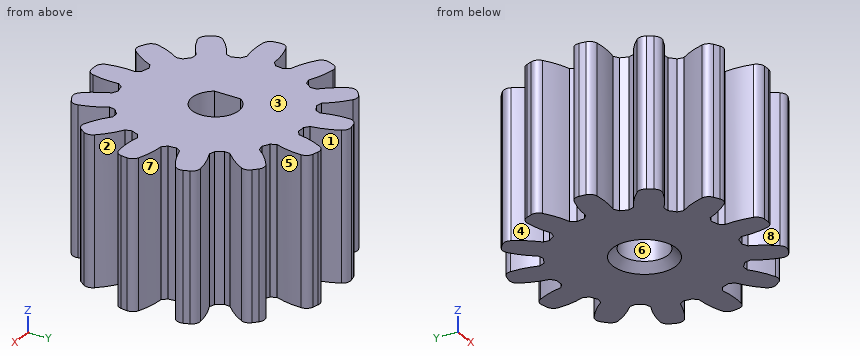
```python
from build123d import *

# Parameters (mm, degrees)
SKETCH1_R           = 15
BOSS_EXTRUDE1_DEPTH = 9
CUT_EXTRUDE1_DEPTH  = 24.043437244
CIRPATTERN1_COUNT   = 13
FILLET1_R           = 1
SKETCH3_R           = 2.85
CUT_EXTRUDE2_DEPTH  = 24
BOSS_EXTRUDE2_DEPTH = 8.5
FILLET3_R           = 1
CHAMFER2_SIZE       = 1


with BuildPart() as part:
    # Sketch1 → Boss-Extrude1 (new, symmetric)
    with BuildSketch(Plane.XY):
        Circle(SKETCH1_R)
    extrude(amount=BOSS_EXTRUDE1_DEPTH, both=True)

    # Sketch2 → Cut-Extrude1 (cut, symmetric)
    with BuildSketch(Plane.XY):
        with BuildLine():
            Line((2.488704723, 14.792104272), (2.488704723, 15.173999235))
            Line((2.488704723, 15.173999235), (-2.614354336, 15.173999235))
            Line((-2.614354336, 15.173999235), (-2.488704723, 14.792104272))
            ThreePointArc((-2.488704723, 14.792104272), (-1.497391845, 12.707607266), (-1.01110734, 10.451203852))
            ThreePointArc((-1.01110734, 10.451203852), (0, 10.5), (1.01110734, 10.451203852))
            ThreePointArc((1.01110734, 10.451203852), (1.497391845, 12.707607266), (2.488704723, 14.792104272))
        make_face()
    cut_extrude1 = extrude(amount=CUT_EXTRUDE1_DEPTH, both=True, mode=Mode.SUBTRACT)

    # CirPattern1: Cut-Extrude1 ×13 about axis
    cirpattern1_axis = Axis((0, 0, 0), (0, 0, 1))
    for i in range(1, CIRPATTERN1_COUNT):
        add(cut_extrude1.rotate(cirpattern1_axis, i * 360 / CIRPATTERN1_COUNT), mode=Mode.SUBTRACT)

    # Fillet1
    fillet1_edges = [part.edges().sort_by_distance(p)[0] for p in [
        (11.67180174, -9.421732544, 0),
        (7.946157272, -12.722365527, 0),
        (14.713364615, -2.918373125, 0),
        (-2.488704723, 14.792104272, 0),
        (12.948350901, -7.572331804, 0),
        (5.956369747, -13.766686582, 0),
        (1.123594773, -14.95785863, 0),
        (2.488704723, 14.792104272, 0),
        (-1.123594773, -14.95785863, 0),
        (-5.956369747, -13.766686582, 0),
        (-12.948350901, -7.572331804, 0),
        (-14.713364615, -2.918373125, 0),
        (-7.946157272, -12.722365527, 0),
        (-11.67180174, -9.421732544, 0),
        (-9.077872212, 11.941199107, 0),
        (-4.670595026, 14.254316613, 0),
        (-13.587408577, 6.354709133, 0),
        (-10.759917741, 10.451036801, 0),
        (-14.984233383, -0.68756812, 0),
        (-14.384272972, 4.253550406, 0),
        (4.670595026, 14.254316613, 0),
        (9.077872212, 11.941199107, 0),
        (10.759917741, 10.451036801, 0),
        (13.587408577, 6.354709133, 0),
        (14.384272972, 4.253550406, 0),
        (14.984233383, -0.68756812, 0),
    ]]
    fillet(fillet1_edges, radius=FILLET1_R)

    # Chamfer1
    # the kernel refuses this chamfer: 0.5 mm, written as the material it adds along each edge
    with BuildSketch(Plane(origin=(7.687254792, -7.152350227, 9), x_dir=(-0.6988462718759633, -0.7152718981513725, 0), z_dir=(0, 0, -1)), Plane(origin=(3.482863191, -9.905537037, 9), x_dir=(-0.9512010678205252, -0.3085717559613855, 0), z_dir=(0, 0, -1)), Plane(origin=(-1.519410394, -10.389484687, 9), x_dir=(-0.9856471623429421, 0.16881845682657493, 0), z_dir=(0, 0, -1)), Plane(origin=(-9.413501753, -4.651449748, 9), x_dir=(-0.42097653940929197, 0.9070715259928386, 0), z_dir=(0, 0, -1)), Plane(origin=(-6.173605368, -8.493326601, 9), x_dir=(-0.7942933703085662, 0.6075343956385179, 0), z_dir=(0, 0, -1)), Plane(origin=(-10.496878331, 0.256018188, 9), x_dir=(0.048780943351376956, 0.998809501139106, 0), z_dir=(0, 0, -1))) as chamfer1_piece_1:
        with BuildLine():
            Line((0.512668458, 0), (-0.025719054, -0.512719416))
            ThreePointArc((-0.025719054, -0.512719416), (-0.009930751, -0.26377362), (0, 0))
            ThreePointArc((0, 0), (0.263582733, -0.00312688), (0.512668458, 0))
        make_face()
    extrude(amount=18)
    with BuildSketch(Plane(origin=(6.173605368, -8.493326601, 9), x_dir=(0.5669781411868423, -0.8237328374031918, 0), z_dir=(0, 0, -1)), Plane(origin=(9.413501753, -4.651449748, 9), x_dir=(0.8848419486421701, -0.4658913241552447, 0), z_dir=(0, 0, -1)), Plane(origin=(1.519410394, -10.389484687, 9), x_dir=(0.11922647441292282, -0.9928670846589006, 0), z_dir=(0, 0, -1)), Plane(origin=(-3.482863191, -9.905537037, 9), x_dir=(-0.3558385408142222, -0.934547448164728, 0), z_dir=(0, 0, -1)), Plane(origin=(-10.130588961, -2.760646175, 9), x_dir=(-0.971256802316475, -0.23803408149669583, 0), z_dir=(0, 0, -1)), Plane(origin=(-7.687254792, -7.152350227, 9), x_dir=(-0.7493852346601237, -0.6621342538136743, 0), z_dir=(0, 0, -1)), Plane(origin=(-10.253127286, 2.263488646, 9), x_dir=(-0.9706251414754602, 0.24059683026952544, 0), z_dir=(0, 0, -1))) as chamfer1_piece_2:
        with BuildLine():
            Line((0.513364071, 0), (-0.025684204, -0.512024677))
            ThreePointArc((-0.025684204, -0.512024677), (-0.010082291, -0.263408394), (0, 0))
            ThreePointArc((0, 0), (0.263939908, -0.003296528), (0.513364071, 0))
        make_face()
    extrude(amount=18)
    with BuildSketch(Plane(origin=(-1.01110734, 10.451203852, 9), x_dir=(-0.12184667616261032, 0.9925489345660113, 0), z_dir=(0, 0, -1)), Plane(origin=(10.130588961, -2.760646175, 9), x_dir=(0.9712568023164747, -0.2380340814966975, 0), z_dir=(0, 0, -1)), Plane(origin=(-5.752207693, 8.784196415, 9), x_dir=(-0.569150362894187, 0.822233461017864, 0), z_dir=(0, 0, -1)), Plane(origin=(-9.175546584, 5.104835441, 9), x_dir=(-0.8860685604921126, 0.46355421053792145, 0), z_dir=(0, 0, -1)), Plane(origin=(3.961625519, 9.723966436, 9), x_dir=(0.35337061566617867, 0.9354834087164272, 0), z_dir=(0, 0, -1)), Plane(origin=(8.026797714, 6.769085497, 9), x_dir=(0.7476349580234212, 0.664109907727115, 0), z_dir=(0, 0, -1)), Plane(origin=(10.253127286, 2.263488646, 9), x_dir=(0.9706251414754612, 0.24059683026952128, 0), z_dir=(0, 0, -1))) as chamfer1_piece_3:
        with BuildLine():
            Line((0.513364071, 0), (-0.025684204, 0.512024677))
            ThreePointArc((-0.025684204, 0.512024677), (-0.010082291, 0.263408394), (0, 0))
            ThreePointArc((0, 0), (0.263939908, 0.003296528), (0.513364071, 0))
        make_face()
    extrude(amount=18)
    with BuildSketch(Plane(origin=(1.01110734, 10.451203852, 9), x_dir=(-0.9974069482855394, 0.07196790612298887, 0), z_dir=(0, 0, -1)), Plane(origin=(-3.961625519, 9.723966436, 9), x_dir=(-0.916605146006636, -0.39979370469550085, 0), z_dir=(0, 0, -1)), Plane(origin=(-8.026797714, 6.769085497, 9), x_dir=(-0.6258201510670891, -0.7799673958047002, 0), z_dir=(0, 0, -1)), Plane(origin=(5.752207693, 8.784196415, 9), x_dir=(-0.8497148387689841, 0.5272425369560002, 0), z_dir=(0, 0, -1)), Plane(origin=(9.175546584, 5.104835441, 9), x_dir=(-0.5073632998643495, 0.8617322565337555, 0), z_dir=(0, 0, -1)), Plane(origin=(10.496878331, 0.256018188, 9), x_dir=(-0.04878094335137992, 0.9988095011391058, 0), z_dir=(0, 0, -1))) as chamfer1_piece_4:
        with BuildLine():
            Line((0.512668458, 0), (-0.025719054, 0.512719416))
            ThreePointArc((-0.025719054, 0.512719416), (-0.009930751, 0.26377362), (0, 0))
            ThreePointArc((0, 0), (0.263582733, 0.00312688), (0.512668458, 0))
        make_face()
    extrude(amount=18)

    # Sketch3 → Cut-Extrude2 (cut)
    with BuildSketch(Plane(origin=(0, 0, -9), x_dir=(-1, 0, 0), z_dir=(0, 0, -1))):
        Circle(SKETCH3_R)
    extrude(amount=-CUT_EXTRUDE2_DEPTH, mode=Mode.SUBTRACT)

    # Sketch5 → Boss-Extrude2 (add)
    with BuildSketch(Plane.XY.offset(9)):
        Polygon((-2.35, 0), (-2.35, 1.61245155), (-2.85, 1.61245155), (-2.85, -1.61245155), (-2.35, -1.61245155), align=None)
    extrude(amount=-BOSS_EXTRUDE2_DEPTH)

    # Fillet3
    # the kernel refuses this fillet: 1 mm, written as the material it takes off along each edge
    with BuildSketch(Plane(origin=(-2.35, -4.11245155, 0.5), x_dir=(-1, 0, 0), z_dir=(0, 1, 0))) as fillet3_piece_1_section:
        with BuildLine():
            CenterArc((FILLET3_R, FILLET3_R), FILLET3_R, 180, 90)
            Line((0, FILLET3_R), (0, 0))
            Line((0, 0), (FILLET3_R, 0))
        make_face()
    fillet3_piece_1 = extrude(amount=8.224903099, mode=Mode.PRIVATE)
    fillet3_piece_1 = fillet3_piece_1 & Plane(origin=(0, 0, 0.5), x_dir=(-1, 0, 0), z_dir=(0, 0, -1)) * Cylinder(2.85, 21, mode=Mode.PRIVATE)
    add(fillet3_piece_1, mode=Mode.SUBTRACT)

    # Chamfer2
    chamfer2_edges = [part.edges().sort_by_distance(p)[0] for p in [
        (2.85, 0, -9),
    ]]
    chamfer(chamfer2_edges, length=CHAMFER2_SIZE)


solid = part.part
```
Read the model definition and answer for the solid it produces. Units are mm, in the model's axes. Face numbers are marked on the shaded views. A direction names the side the tool comes from. Give positions to 0.01 mm unless a question says otherwise; leave off trailing zeros. Order: outer loops, then holes, each group sorted by start corner. A loop starts at its lowest first (then second) coordinate and runs counter-clockwise, first axis right, second up.
(1) Straight lines are drawn through the part: L1, parallel to Y at x = -12.5, z = 4.5; L2, parallel to X at y = -10.5, z = 0.5; L3, parallel to X at y = 9.5, z = -1.5. For each, find the intervals that lie inside material, in ascending order.
(2) For the marked faces 4, 5, 6, 7 and 8, determine the directions among +Z, -Z, +X, -X, +Y, -Y from which every point of the face is accessible in a straight line to the end or side of a thin tool.
(3) Find section A-A (x = 0). Give the vertices of the cut face in (y, z).
(4) For a pull along Y with two mould halves and no side action, classify the marked faces 1, 2 and 3 as released by +Y, released by -Y, zero draft, split by the parting line, or undercut.
(5) Given pin 1 (4.5 mm diameter, centred on x = 0, y = 0, fed in from +Z); pin 2 (10 mm diameter, centred on y = 6.5, z = 4.5, fed in from +X); pin 3 (1.5 mm diameter, centred on x = -6, z = -7, fed in from +Y), each flat-ended and moving along its own axis, determine where each tip first touches the part or whether it passes through.
Result sheet:
1. L1: y = -8.29 to -7.02, -3.11 to 0.1, 3.05 to 6.25
1. L2: x = -7.3 to -3.71, -1.88 to 1.88, 3.71 to 7.3
1. L3: x = -10.29 to -6.27, -4.47 to 4.47, 6.27 to 10.29
2. face 4: +Z, -Z, -X
2. face 5: +Z, -Z
2. face 6: -Z
2. face 7: +Z, -Z, +X
2. face 8: +Z, -Z, -Y
3. outline: (-15, -9) - (-3.85, -9) - (-2.85, -8) - (-2.85, 9) - (-15, 9) - close; (2.85, -8) - (3.85, -9) - (10.5, -9) - (10.5, 9) - (2.85, 9) - close
4. face 1: released by +Y
4. face 2: undercut
4. face 3: zero draft
5. pin 1: passes through
5. pin 2: stops at x = 14.21
5. pin 3: stops at y = 10.07
